from build123d import *

# Parameters (mm, degrees)
SKETCH_3_R      = 1.5
SKETCH_3_R_2    = 5
SKETCH_3_W      = 3
SKETCH_3_H      = 10
EXTRUDE_1_DEPTH = 4
FILLET_2_R      = 5
FILLET_4_R      = 200
FILLET_5_R      = 200
FILLET_8_R      = 200
FILLET_9_R      = 200
FILLET_START    = -1
FILLET_10_DEPTH = 6
FILLET_11_DEPTH = 6
FILLET_13_R     = 200
FILLET_1_R      = 40


with BuildPart() as part:
    # Эскиз3 → Бобышка-Вытянуть1 (new body)
    with BuildSketch(Plane(origin=(0, 0, 0), x_dir=(1, 0, 0), z_dir=(0, 1, 0))):
        with BuildLine():
            Line((18.75, 35.128113741), (131.25, 35.128113741))
            Line((131.25, 35.128113741), (150, 46.837484988))
            ThreePointArc((150, 46.837484988), (166.583269132, 25.980762114), (172.5, 0))
            Line((172.5, 0), (162.5, -45))
            Line((162.5, -45), (147.5, -105))
            Line((147.5, -105), (150, -150))
            Line((150, -150), (172.5, -220))
            Line((172.5, -220), (172.5, -310))
            Line((172.5, -310), (135, -310))
            Line((135, -310), (75, -290))
            Line((75, -290), (15, -310))
            Line((15, -310), (-22.5, -310))
            Line((-22.5, -310), (-22.5, -220))
            Line((-22.5, -220), (0, -150))
            Line((0, -150), (2.5, -105))
            Line((2.5, -105), (-12.5, -45))
            Line((-12.5, -45), (-22.5, 0))
            ThreePointArc((-22.5, 0), (-16.583269132, 25.980762114), (0, 46.837484988))
            Line((0, 46.837484988), (18.75, 35.128113741))
        make_face()
        with Locations(Location((150, 0, 0), (0, 0, 270))):
            Circle(SKETCH_3_R, mode=Mode.SUBTRACT)
        with Locations(Location((0, 0, 0), (0, 0, 270))):
            Circle(SKETCH_3_R, mode=Mode.SUBTRACT)
        with Locations(Location((150, -270, 0), (0, 0, 270))):
            Circle(SKETCH_3_R_2, mode=Mode.SUBTRACT)
        with Locations(Location((0, -270, 0), (0, 0, 270))):
            Circle(SKETCH_3_R_2, mode=Mode.SUBTRACT)
        with Locations(Location((-6.8, -262.3, 0), (0, 0, 270))):
            Circle(SKETCH_3_R, mode=Mode.SUBTRACT)
        with Locations(Location((6.8, -262.3, 0), (0, 0, 270))):
            Circle(SKETCH_3_R, mode=Mode.SUBTRACT)
        with Locations(Location((-6.8, -277.7, 0), (0, 0, 270))):
            Circle(SKETCH_3_R, mode=Mode.SUBTRACT)
        with Locations(Location((6.8, -277.7, 0), (0, 0, 270))):
            Circle(SKETCH_3_R, mode=Mode.SUBTRACT)
        with Locations(Location((143.2, -262.3, 0), (0, 0, 270))):
            Circle(SKETCH_3_R, mode=Mode.SUBTRACT)
        with Locations(Location((156.8, -262.3, 0), (0, 0, 270))):
            Circle(SKETCH_3_R, mode=Mode.SUBTRACT)
        with Locations(Location((143.2, -277.7, 0), (0, 0, 270))):
            Circle(SKETCH_3_R, mode=Mode.SUBTRACT)
        with Locations(Location((156.8, -277.7, 0), (0, 0, 270))):
            Circle(SKETCH_3_R, mode=Mode.SUBTRACT)
        with Locations(Location((61.5, 4.5, 0), (0, 0, 270))):
            Circle(SKETCH_3_R, mode=Mode.SUBTRACT)
        with Locations(Location((61.5, -4.5, 0), (0, 0, 270))):
            Circle(SKETCH_3_R, mode=Mode.SUBTRACT)
        with Locations(Location((108.5, -4.5, 0), (0, 0, 90))):
            Circle(SKETCH_3_R, mode=Mode.SUBTRACT)
        with Locations(Location((108.5, 4.5, 0), (0, 0, 90))):
            Circle(SKETCH_3_R, mode=Mode.SUBTRACT)
        with Locations(Location((35, -36, 0), (0, 0, 270))):
            Circle(SKETCH_3_R, mode=Mode.SUBTRACT)
        with Locations(Location((115, -36, 0), (0, 0, 270))):
            Circle(SKETCH_3_R, mode=Mode.SUBTRACT)
        with Locations(Location((115, -156, 0), (0, 0, 270))):
            Circle(SKETCH_3_R, mode=Mode.SUBTRACT)
        with Locations(Location((35, -156, 0), (0, 0, 270))):
            Circle(SKETCH_3_R, mode=Mode.SUBTRACT)
        with Locations(Location((56.615223689, -196.934776311, 0), (0, 0, 270))):
            Circle(SKETCH_3_R, mode=Mode.SUBTRACT)
        with Locations(Location((93.384776311, -196.934776311, 0), (0, 0, 270))):
            Circle(SKETCH_3_R, mode=Mode.SUBTRACT)
        with Locations(Location((93.384776311, -160.165223689, 0), (0, 0, 270))):
            Circle(SKETCH_3_R, mode=Mode.SUBTRACT)
        with Locations(Location((56.615223689, -160.165223689, 0), (0, 0, 270))):
            Circle(SKETCH_3_R, mode=Mode.SUBTRACT)
        with Locations(Location((56.615223689, -50.134776311, 0), (0, 0, 270))):
            Circle(SKETCH_3_R, mode=Mode.SUBTRACT)
        with Locations(Location((93.384776311, -50.134776311, 0), (0, 0, 270))):
            Circle(SKETCH_3_R, mode=Mode.SUBTRACT)
        with Locations(Location((93.384776311, -13.365223689, 0), (0, 0, 270))):
            Circle(SKETCH_3_R, mode=Mode.SUBTRACT)
        with Locations(Location((56.615223689, -13.365223689, 0), (0, 0, 270))):
            Circle(SKETCH_3_R, mode=Mode.SUBTRACT)
        Polygon((65, 10), (65, 0), (65, -10), (75, -10), (105, -10), (105, 10), (85, 10), align=None, mode=Mode.SUBTRACT)
        with Locations((48.5, -25)):
            Rectangle(SKETCH_3_W, SKETCH_3_H, mode=Mode.SUBTRACT)
        with Locations((101.5, -25)):
            Rectangle(SKETCH_3_W, SKETCH_3_H, mode=Mode.SUBTRACT)
    extrude(amount=EXTRUDE_1_DEPTH)

    # Скругление2
    fillet_2_edges = [part.edges().sort_by_distance(p)[0] for p in [
        (-22.5, 2, 0),
    ]]
    fillet(fillet_2_edges, radius=FILLET_2_R)

    # Скругление4
    # the kernel refuses this fillet: 200 mm, written as the material it takes off along each edge
    with BuildSketch(Plane(origin=(-12.5, -6.577808748, 45), x_dir=(-0.21693045781865417, 0, -0.9761870601839532), z_dir=(0, 1, 0))) as fillet_4_piece_1:
        with BuildLine():
            CenterArc((FILLET_4_R * 0.0131556174964, -FILLET_4_R), FILLET_4_R, 90, 1.507435759)
            Line((-FILLET_4_R * 0.0131510645918, -FILLET_4_R * 0.000346080647153), (0, 0))
            Line((0, 0), (FILLET_4_R * 0.0131556174964, 0))
        make_face()
    extrude(amount=17.155617496, mode=Mode.SUBTRACT)

    # Скругление5
    fillet_5_edges = [part.edges().sort_by_distance(p)[0] for p in [
        (2.5, 2, 105),
    ]]
    fillet(fillet_5_edges, radius=FILLET_5_R)

    # Скругление8
    fillet_8_edges = [part.edges().sort_by_distance(p)[0] for p in [
        (-22.5, 2, 220),
    ]]
    fillet(fillet_8_edges, radius=FILLET_8_R)

    # Скругление9
    fillet_9_edges = [part.edges().sort_by_distance(p)[0] for p in [
        (172.5, 2, 220),
    ]]
    fillet(fillet_9_edges, radius=FILLET_9_R)

    # Скругление10: read off the stored shape, not the designer's step
    # Скругление10 outline → Скругление10 (cut)
    with BuildSketch(Plane(origin=(0, 0, 0), x_dir=(1, 0, 0), z_dir=(0, 1, 0)).offset(FILLET_START)):
        with BuildLine():
            Line((-22.5, -310), (8.288353461, -310))
            add(Edge.make_bspline(
                [(8.288353461, -310), (-29.099560998, -310), (-21.57252534, -232.114186903)],
                knots=[0, 0, 0, 1, 1, 1], degree=2, weights=[1, 0.672237395, 1]))
            ThreePointArc((-21.57252534, -232.114186903), (-22.267996771, -241.722392301), (-22.5, -251.352940882))
            Line((-22.5, -251.352940882), (-22.5, -310))
        make_face()
    extrude(amount=FILLET_10_DEPTH, mode=Mode.SUBTRACT)

    # Скругление11: read off the stored shape, not the designer's step
    # Скругление11 outline → Скругление11 (cut)
    with BuildSketch(Plane(origin=(0, 0, 0), x_dir=(1, 0, 0), z_dir=(0, 1, 0)).offset(FILLET_START)):
        with BuildLine():
            ThreePointArc((172.5, -251.352940882), (172.281100603, -241.998164461), (171.624881581, -232.663865588))
            add(Edge.make_bspline(
                [(171.624881581, -232.663865588), (178.883345855, -310), (146.734271383, -310)],
                knots=[0, 0, 0, 1, 1, 1], degree=2, weights=[1, 0.673258726, 1]))
            Line((146.734271383, -310), (172.5, -310))
            Line((172.5, -310), (172.5, -251.352940882))
        make_face()
    extrude(amount=FILLET_11_DEPTH, mode=Mode.SUBTRACT)

    # Скругление13
    fillet_13_edges = [part.edges().sort_by_distance(p)[0] for p in [
        (147.5, 2, 105),
    ]]
    fillet(fillet_13_edges, radius=FILLET_13_R)

    # Скругление1
    fillet_1_edges = [part.edges().sort_by_distance(p)[0] for p in [
        (18.75, 2, -35.128113741),
        (131.25, 2, -35.128113741),
    ]]
    fillet(fillet_1_edges, radius=FILLET_1_R)


solid = part.part
Source: CAD feature listing. Evaluate the final solid. Frame: model axes, mm. A direction names the side the tool comes from. Round coordinates to 2 decimals unless told otherwise and drop trailing zeros. Loops run counter-clockwise (first coordinate to the right, second up) from the corner with the lowest first, then second, coordinate; pieces in that order, holes last. Notation, with made-up numbers: M 88.25,58.25 L 112.25,58.25 A19 ccw 112.25,63.25 Z; hole C 51.5,-25.75 d3. An arc over 180 degrees is marked long. Return JSON: item names as keys, results as strings. Group by question number.
1. Section query C-C on z = 182. Output: boundary loops of the cut face in (x, y).
2. Section query A-A on y = 2.55. State how many separate pieces and enclosed holes the cut face has, and give its area (3 significant figures).
3. Material intervals for line 1 along X through (y, z) = (2.15, -4.5); line 2 along X through (y, z) = (1, 270); line 3 along X through (y, z) = (1.5, 156), sorted ascending. Write a range as from..to.
4. Pin query (flat end, axial travel): pin 1 (2 mm diameter, centred on y = 2, z = 5, fed in from +X); pin 2 (1.5 mm diameter, centred on x = 49, y = 1.5, fed in from -Z). Return the tip coordinate at first contact, or that it passes through.
5. Mould query, pull axis X, two halves, no side actions, for faces 4 (the face through (1.5, 1.97, 274.77)), 5 (the face through (158.725, 1.972, 60.1)), 6 (the face through (76, 4, 129)). Classes: released by +X, released by -X, zero draft, split by the parting line, or undercut.
6. Section query B-B on x = 21. Output: boundary loops of the cut face in (y, z).
7. Reachability of faces 1 (the face through (-17.66, 1.97, 21.78)), 2 (the face through (156.36, 1.97, 169.79)), 3 (the face through (45, 2, 300)) from +Z, -Z, +X, -X, +Y, -Y: full face, straight path, thin tool, end or side. Return the list, or none.
Checks:
{
 "1": {"outline": "M -10.29,0 L 160.29,0 L 160.29,4 L -10.29,4 Z"},
 "2": {"separate pieces": "1", "enclosed holes": "31", "area": "58,000 mm²"},
 "3": {"line 1": "x = -22.33..60, 63..65, 105..107, 110..172.33", "line 2": "x = -20.23..-5, 5..145, 155..170.9", "line 3": "x = -1.93..33.5, 36.5..113.5, 116.5..151.93"},
 "4": {"pin 1": "stops at x = 171.61", "pin 2": "stops at z = -35.13"},
 "5": {"face 4": "undercut", "face 5": "released by +X", "face 6": "zero draft"},
 "6": {"outline": "M 0,-36.2 L 4,-36.2 L 4,308 L 0,308 Z"},
 "7": {"face 1": "-X, +Y, -Y", "face 2": "+X, +Y, -Y", "face 3": "+Z, +Y, -Y"}
}
